```python
from build123d import *

# Parameters (mm, degrees)
F1_DEPTH = 19.05
F2_R     = 1.5875
F3_DEPTH = 12.7
F4_DEPTH = 19.05
F5_DEPTH = 19.05
F6_DEPTH = 19.05


with BuildPart() as f1:
    # F0 (on Front) → F1 (new body)
    with BuildSketch(Plane.XZ):
        with BuildLine():
            Line((120.142, 155.7741917981), (0, 155.7741917981))
            Line((0, 155.7741917981), (-120.142, 155.7741917981))
            Line((-120.142, 155.7741917981), (-120.142, 143.0741917981))
            Line((-120.142, 143.0741917981), (-227.8642566605, -116.5812388062))
            Line((-227.8642566605, -116.5812388062), (-120.142, -116.5812388062))
            ThreePointArc((-120.142, -116.5812388062), (0, 7.246479044), (120.142, -116.5812388062))
            Line((120.142, -116.5812388062), (227.8642566605, -116.5812388062))
            Line((227.8642566605, -116.5812388062), (120.142, 143.0741917981))
            Line((120.142, 143.0741917981), (120.142, 155.7741917981))
        make_face()
    extrude(amount=F1_DEPTH)

    # F2 (on Front) → F3 (cut)
    with BuildSketch(Plane.XZ):
        Polygon((-9.652, 29.7901917981), (0, 29.7901917981), (9.652, 29.7901917981), (9.652, 155.7741917981), (0, 155.7741917981), (-9.652, 155.7741917981), align=None)
        with Locations((0, 62.8101917981)):
            Circle(F2_R, mode=Mode.SUBTRACT)
        with Locations((0, 93.7981917981)):
            Circle(F2_R, mode=Mode.SUBTRACT)
        with Locations((0, 124.2781917981)):
            Circle(F2_R, mode=Mode.SUBTRACT)
    extrude(amount=F3_DEPTH, mode=Mode.SUBTRACT)

    # F4 (cut): a face of the model
    f4_faces = [f1.faces().sort_by_distance(p)[0] for p in [
        (0, 0, 124.2781917981),
    ]]
    extrude(f4_faces, amount=-F4_DEPTH, mode=Mode.SUBTRACT)

    # F5 (cut): a face of the model
    f5_faces = [f1.faces().sort_by_distance(p)[0] for p in [
        (0, 0, 93.7981917981),
    ]]
    extrude(f5_faces, amount=-F5_DEPTH, mode=Mode.SUBTRACT)

    # F6 (cut): a face of the model
    f6_faces = [f1.faces().sort_by_distance(p)[0] for p in [
        (0, 0, 62.8101917981),
    ]]
    extrude(f6_faces, amount=-F6_DEPTH, mode=Mode.SUBTRACT)


solid = f1.part
```
Here's how the part is built. I have some questions about the finished solid (model axes, mm). A direction names the side the tool comes from. Give positions to 0.01 mm unless a question says otherwise; leave off trailing zeros. Loops run counter-clockwise (first coordinate to the right, second up) from the corner with the lowest first, then second, coordinate; pieces in that order, holes last. Notation, with made-up numbers: (17, 62) -> (24, 62) arc R23 ccw to (24, 99) -> close; hole circle Ø1 at (-36, 59). An arc over 180 degrees is marked (long way). Use one line per item in the form item = value. Start each with the question number.
1) For P1, Ø4, axis at y = -13, z = 146.5, coming from the -X side; P2, Ø4, axis at y = -6, z = -35, coming from the -X side; P3, Ø1.5, axis at y = -6, z = 5, coming from the -X side; P4, Ø3, axis at x = 0, z = 62.81, coming from the -Y side, each with a flat end and sliding along its axis, tell me the tip position at first contact or that it passes through.
2) Imagine slicing it at B-B (z = 80). Please give me the cut outline in (x, y).
3) Which directions (+Z, -Z, +X, -X, +Y, -Y) give clear straight access to the entire face, cutting with the end or side of a thin tool? Please do faces 1 (the face through (173, -9, -116.581)), 2 (the face through (-2, -12.7, 94)), 3 (the face through (120.142, -9, 149)).
4) Please list where these lines run through material, in increasing order: line 1 along Z through (x, y) = (0, -16.25); line 2 along X through (y, z) = (-4.5, -68.5); line 3 along X through (y, z) = (-4.75, -46).
5) Imagine slicing it at A-A (y = -7). Please give me the cut outline in (x, z).
6) Imagine slicing it at C-C (x = -199). Please give me the cut outline in (y, z), then the cut area to 3 significant figures.
7) Thinking about a two-plate mould opening in X: for faces 4 (the face through (-120.142, -9, 150)), 5 (the face through (-2.694, -9.392, 7.216)), 6 (the face through (-175, -9, -116.581)), which applies, +X half, -X half, draft (parallel to the pull), parting line (faces both ways), or undercut?
Check values:
q1.P1 = -120.14
q1.P2 = -194.85
q1.P3 = -177.74
q1.P4 = through
q2.outline = (-146.31, -19.05) -> (146.31, -19.05) -> (146.31, 0) -> (9.65, 0) -> (9.65, -12.7) -> (-9.65, -12.7) -> (-9.65, 0) -> (-146.31, 0) -> close
q3.face_1 = -Z, +X, -X, +Y, -Y
q3.face_2 = +Z, +Y
q3.face_3 = +Z, +X, +Y, -Y
q4.line_1 = 7.25 to 61.22, 64.4 to 92.21, 95.39 to 122.69, 125.87 to 155.77
q4.line_2 = -207.92 to -111.68, 111.68 to 207.92
q4.line_3 = -198.58 to -99.82, 99.82 to 198.58
q5.outline = (-227.86, -116.58) -> (-120.14, -116.58) arc R120.2 cw (long way) to (120.14, -116.58) -> (227.86, -116.58) -> (120.14, 143.07) -> (120.14, 155.77) -> (9.65, 155.77) -> (9.65, 29.79) -> (-9.65, 29.79) -> (-9.65, 155.77) -> (-120.14, 155.77) -> (-120.14, 143.07) -> close
q6.outline = (-19.05, -116.58) -> (0, -116.58) -> (0, -47.01) -> (-19.05, -47.01) -> close
q6.area = 1,330 mm^2
q7.face_4 = -X half
q7.face_5 = undercut
q7.face_6 = draft
